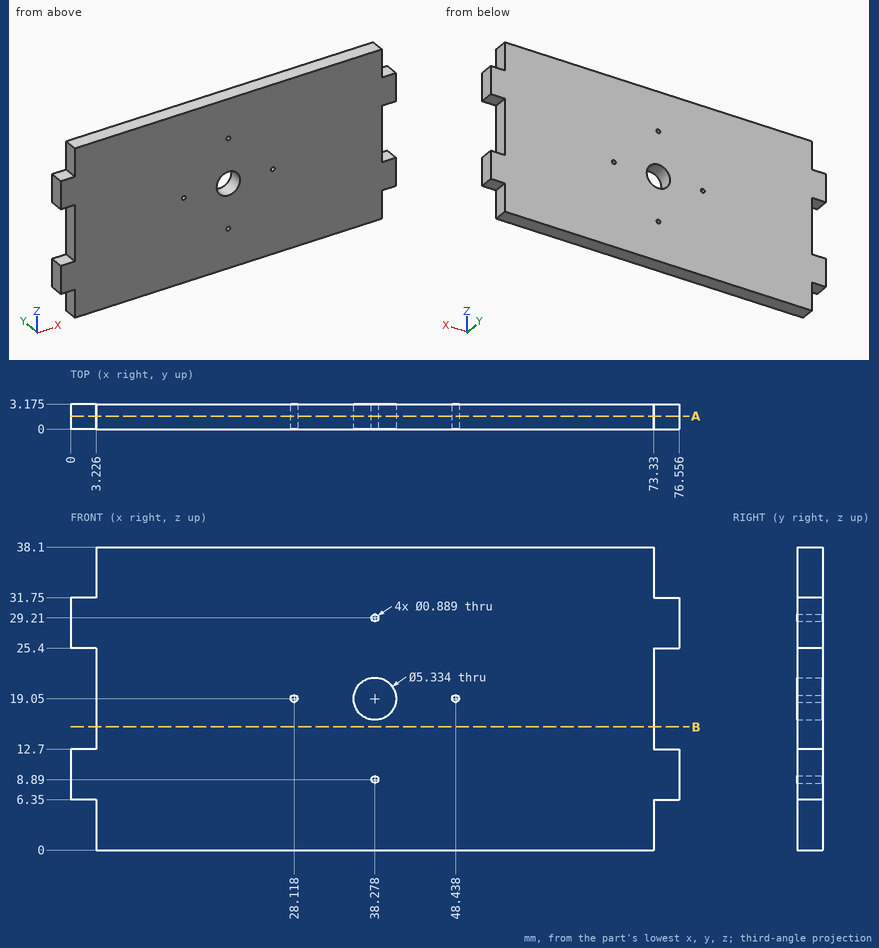
Could you check a few things on this drawing? It's one solid part, dimensions in mm from its lowest x, y, z. Round coordinates to 2 decimals unless told otherwise and drop trailing zeros. Order: outer loops, then holes, each group sorted by start corner. A loop starts at its lowest first (then second) coordinate and runs counter-clockwise, first axis right, second up. Notation, with made-up numbers: M 0.25,-18.5 L 57.25,-18.5 A29 cw 57.25,2.5 Z; hole C 62,79 d1. An arc over 180 degrees is marked long. Return JSON: item names as keys, results as strings. Group by question number.
1. If we section it at B-B on z = 15.5: List the corners of the cut face in (x, y) for me (1 decimal).
2. Please list where these lines run through material, in increasing order: probe 1 along X at (y, z) = (1.45, 19.05) (1 decimal); probe 2 along X at (y, z) = (2.2, 16) (1 decimal); probe 3 along X at (y, z) = (1.6, 18) (1 decimal).
3. I'm going to push flat-ended pins straight in: pin 1 Ø8.5 at (x, z) = (38.28, 19.05) entering from -Y; pin 2 Ø1.6 at (x, y) = (75, 2) entering from -Z; pin 3 Ø1 at (y, z) = (1.5, 21.5) entering from +X; pin 4 Ø1 at (y, z) = (2, 36) entering from -X. Where does each tip first touch, or does it pass through?
4. If we section it at A-A on y = 1.65: State how many separate pieces and enclosed holes the cut face has, then the cut area to 3 significant figures.
Reply:
{
 "1": {"outline": "M 3.2,0 L 73.3,0 L 73.3,3.2 L 3.2,3.2 Z"},
 "2": {"probe 1": "3.2 to 27.7, 28.6 to 35.6, 40.9 to 48, 48.9 to 73.3", "probe 2": "3.2 to 73.3", "probe 3": "3.2 to 35.8, 40.7 to 73.3"},
 "3": {"pin 1": "y = 0", "pin 2": "z = 6.35", "pin 3": "x = 73.33", "pin 4": "x = 3.23"},
 "4": {"separate pieces": "1", "enclosed holes": "5", "area": "2,730 mm^2"}
}
